Input: part model. Units: mm. Frame: model coordinates. Coordinates: 2 decimals unless noted, no trailing zeros. Write each loop counter-clockwise with the first axis right and the second up, starting at its lowest first coordinate (ties: lowest second). Pieces come first, ordered by that corner, then holes. Notation, with made-up numbers: M 89.25,51.5 L 139.25,51.5 A19 cw 139.25,72.5 Z; hole C 38.25,89 d7. An arc over 180 degrees is marked long. Write each question's results on one line, items separated by ' | '. Start each with the question number.
1. Section query D-D, the plane x = -73. Output: boundary loops of the cut face in (y, z), and give its area (3 significant figures).
2. Ray query, probe 1 along Y at (x, z) = (31, 1.15); probe 2 along X at (y, z) = (-1, 3.7); probe 3 along X at (y, z) = (-40, 2.85). Return the intervals inside material, ascending.
3. First-contact query: pin 1 (2 mm diameter, centred on x = 33.5, z = 3, fed in from +Y); pin 2 (1 mm diameter, centred on y = -32, z = 1.5, fed in from -X). Flat tips, straight axial feed; report the tip coordinate or a pass-through.
4. Section query B-B, the plane y = -6. Output: boundary loops of the cut face in (x, z), and give its area (3 significant figures).
5. Section query A-A, the plane x = -33. Output: boundary loops of the cut face in (y, z).
6. Section query C-C, the plane z = 3.15. Count the separate pieces of the cut face and the enclosed holes in it, and give its area (3 significant figures).
```python
from build123d import *

# Parameters (mm, degrees)
BOSS_EXTRU_1_DEPTH         = 4
ESQUISSE2_W                = 4
ESQUISSE2_H                = 30
ENL_V_MAT_EXTRU_1_DEPTH    = 4
R_P_TITION_LIN_AIRE1_COUNT = 2
R_P_TITION_LIN_AIRE1_PITCH = 50
ESQUISSE3_W                = 25
ESQUISSE3_H                = 4
ESQUISSE3_W_2              = 40
ENL_V_MAT_EXTRU_2_DEPTH    = 4
D_GAGEMENT_M31_D           = 3.4
ESQUISSE9_W                = 250
ESQUISSE9_H                = 4
BOSS_EXTRU_2_DEPTH         = 5
ESQUISSE10_R               = 1.7
ENL_V_MAT_EXTRU_3_DEPTH    = 10


with BuildPart() as part:
    # Esquisse1 → Boss.-Extru.1 (new body)
    with BuildSketch(Plane.XY):
        Polygon((-8.256647574, 32.690679855), (-4.256647574, 32.690679855), (118.743352426, -83.309320145), (118.743352426, -87.309320145), (-131.256647574, -87.309320145), (-131.256647574, -83.309320145), align=None)
    extrude(amount=BOSS_EXTRU_1_DEPTH)

    # Esquisse2 → Enlèv. mat.-Extru.1 (cut)
    with BuildSketch(Plane.XY.offset(4)):
        with Locations((-6.256647574, -2.309320145)):
            Rectangle(ESQUISSE2_W, ESQUISSE2_H)
    enl_v_mat_extru_1 = extrude(amount=-ENL_V_MAT_EXTRU_1_DEPTH, mode=Mode.SUBTRACT)

    # Répétition linéaire1: Enlèv. mat.-Extru.1 ×2
    with Locations(*[(0, -i * R_P_TITION_LIN_AIRE1_PITCH, 0) for i in range(1, R_P_TITION_LIN_AIRE1_COUNT)]):
        add(enl_v_mat_extru_1, mode=Mode.SUBTRACT)

    # Esquisse3 → Enlèv. mat.-Extru.2 (cut)
    with BuildSketch(Plane.XY.offset(4)):
        with Locations((-118.756647574, -85.309320145)):
            Rectangle(ESQUISSE3_W, ESQUISSE3_H)
        with Locations((33.743352426, -85.309320145)):
            Rectangle(ESQUISSE3_W_2, ESQUISSE3_H)
        with Locations((-46.256647574, -85.309320145)):
            Rectangle(ESQUISSE3_W_2, ESQUISSE3_H)
        with Locations((113.743352426, -85.309320145)):
            Rectangle(ESQUISSE3_W_2, ESQUISSE3_H)
    extrude(amount=-ENL_V_MAT_EXTRU_2_DEPTH, mode=Mode.SUBTRACT)

    # Dégagement M31 (through all)
    with Locations(Plane.XY.offset(4)):
        with Locations((-6.256647574, 22.690679855), (-6.256647574, -27.309320145), (-6.256647574, -77.309320145), (-6.256647574, -85.309320145), (-86.256647574, -85.309320145), (73.743352426, -85.309320145)):
            Hole(D_GAGEMENT_M31_D / 2)

    # Esquisse9 → Boss.-Extru.2 (add)
    with BuildSketch(Plane.XZ.offset(87.309320145)):
        with Locations((-6.256647574, 2)):
            Rectangle(ESQUISSE9_W, ESQUISSE9_H)
    extrude(amount=BOSS_EXTRU_2_DEPTH)

    # Esquisse10 → Enlèv. mat.-Extru.3 (cut)
    with BuildSketch(Plane(origin=(-276.256647574, 4.324322261, 4), x_dir=(1, 0, 0), z_dir=(0, 0, 1))):
        with Locations((308.5, -31.633642405)):
            Circle(ESQUISSE10_R)
    extrude(amount=-ENL_V_MAT_EXTRU_3_DEPTH, mode=Mode.SUBTRACT)


solid = part.part
```
Answer:
1) outline: M -92.31,0 L -28.37,0 L -28.37,4 L -92.31,4 Z | area: 256 mm^2
2) probe 1: -92.31 to -87.31, -83.31 to -28.47, -26.15 to -0.56 | probe 2: -43.98 to -8.26, -4.26 to 31.47 | probe 3: -85.33 to -8.26, -4.26 to 72.82
3) pin 1: y = -1.97 | pin 2: x = -77.38
4) outline: M -49.28,0 L -8.26,0 L -8.26,4 L -49.28,4 Z; M -4.26,0 L 36.77,0 L 36.77,4 L -4.26,4 Z | area: 328 mm^2
5) outline: M -92.31,0 L -87.31,0 L -87.31,4 L -92.31,4 Z; M -83.31,0 L 9.36,0 L 9.36,4 L -83.31,4 Z
6) separate pieces: 1 | enclosed holes: 11 | area: 16,200 mm^2
